The listing builds one solid part. Answer for the finished solid, in the listing's coordinates (mm). A direction names the side the tool comes from. Coordinates: 2 decimals unless noted, no trailing zeros. Loops run counter-clockwise (first coordinate to the right, second up) from the corner with the lowest first, then second, coordinate; pieces in that order, holes last. Notation, with made-up numbers: (-26, 76.25) - (17, 76.25) arc R21 ccw to (17, 109.25) - close; hole circle Ø2 at (-24, 14.25). An arc over 180 degrees is marked (long way). Return JSON: item names as keys, results as strings. Group by question number.
1. The mould has two halves that part along Z. Classify faces 1 (the face through (30, 0, 4.765)), 2 (the face through (0, 0, -7)), 3 (the face through (60, 0, 0)), 4 (the face through (31.9, -11.4, 2.5)): pulls with the +Z half, pulls with the -Z half, needs draft (parallel to the pull), parting line crosses it, or undercut.
2. Section C-C (x = 55.5) is taken. Write down the section's boundary in (y, z) (3 decimals), and give its area (3 significant figures).
3. Section B-B (x = 63) is taken. Write down the section's boundary in (y, z).
4. Which of the six approach directions +Z, -Z, +X, -X, +Y, -Y give full straight-line access (tool end or side, diameter ignored) to faces 5 (the face through (70, 0, 0)), 6 (the face through (30, -7.53, 0))?
5. Each of these flat-tipped pins is pushed along its axis until it touches: P1, Ø5, axis at x = 18, y = -5, coming from the -Z side; P2, Ø8, axis at x = 32.5, y = -8, coming from the +Z side; P3, Ø10.5, axis at x = 39.5, z = 0.5, coming from the -Y side; P4, Ø7.5, axis at y = -0.5, z = 1.5, coming from the -X side. Where does it stop, or does it pass through?
6. Find the intervals of material crossed by line 1 along Z through (x, y) = (7, 0.25) (3 decimals); line 2 along Y through (x, z) = (41, 1.75); line 3 along X through (y, z) = (-5, 2.25), in increasing order.
7. Section A-A (x = 45.5) is taken. Write down the section's boundary in (y, z) (3 decimals).
```python
from build123d import *

# Parameters (mm, degrees)
SZKIC1_R                    = 10
DODANIE_WYCI_GNI_CIE1_DEPTH = 70
DODANIE_WYCI_GNI_CIE1_DRAFT = -3
SZKIC2_W                    = 9.53
SZKIC2_H                    = 15.06
WYTNIJ_WYCI_GNI_CIE1_DEPTH  = 60


with BuildPart() as part:
    # Szkic1 → Dodanie-wyciągnięcie1 (with draft: the straight prism first)
    with BuildSketch(Plane(origin=(0, 0, 0), x_dir=(0, 0, -1), z_dir=(1, 0, 0))):
        Circle(SZKIC1_R)
    extrude(amount=DODANIE_WYCI_GNI_CIE1_DEPTH)
    # Dodanie-wyciągnięcie1: the draft: its side faces are tilted about the plane it starts from
    dodanie_wyci_gni_cie1_sides = [part.faces().sort_by_distance(p)[0] for p in [
        (35, 0, 10),
    ]]
    draft(dodanie_wyci_gni_cie1_sides, Plane(origin=(0, 0, 0), x_dir=(0, 0, -1), z_dir=(1, 0, 0)), DODANIE_WYCI_GNI_CIE1_DRAFT)

    # Zaokrąglenie1
    # a fillet whose section is not a circle: 5 mm, written as the material it takes off along each edge
    with BuildSketch(Plane(origin=(70, 0, 0), x_dir=(0, 0, -1), z_dir=(0, -1, 0))) as zaokr_glenie1_piece_1:
        with BuildLine():
            Bezier((13.392791597, -5.261679781), (13.66854455, 0), (8.399643923, 0), weights=[1, 0.344177288, 1])
            Line((8.399643923, 0), (13.66854455, 0))
            Line((13.66854455, 0), (13.392791597, -5.261679781))
        make_face()
    revolve(axis=Axis((70, 0, 0), (1, 0, 0)), mode=Mode.SUBTRACT)

    # Szkic2 → Wytnij-wyciągnięcie1 (cut)
    with BuildSketch(Plane.ZY):
        Rectangle(SZKIC2_W, SZKIC2_H)
    extrude(amount=-WYTNIJ_WYCI_GNI_CIE1_DEPTH, mode=Mode.SUBTRACT)


solid = part.part
```
The answers:
{
 "1": {"face 1": "undercut", "face 2": "needs draft", "face 3": "undercut", "face 4": "parting line crosses it"},
 "2": {"outline": "circle Ø25.817 at (0, 0); hole (-7.53, -4.765) - (7.53, -4.765) - (7.53, 4.765) - (-7.53, 4.765) - close", "area": "380 mm2"},
 "3": {"outline": "circle Ø26.6 at (0, 0)"},
 "4": {"face 5": "+Z, -Z, +X, +Y, -Y", "face 6": "-X"},
 "5": {"P1": "stops at z = -10.67", "P2": "stops at z = 11.02", "P3": "stops at y = -12.34", "P4": "stops at x = 0"},
 "6": {"line 1": "z = -10.364 to -4.765, 4.765 to 10.364", "line 2": "y = -12.02 to -7.53, 7.53 to 12.02", "line 3": "x = 60 to 70"},
 "7": {"outline": "circle Ø24.769 at (0, 0); hole (-7.53, -4.765) - (7.53, -4.765) - (7.53, 4.765) - (-7.53, 4.765) - close"}
}
